from build123d import *

# Parameters (mm, degrees)
SKETCH1_W                      = 19.05
SKETCH1_H                      = 19.05
SKETCH1_W_2                    = 15.875
SKETCH1_H_2                    = 15.875
TUBE_DEPTH                     = 758.9266
SKETCH2_R                      = 2.8956
SIDE_WALL_HOLES_DEPTH          = 20.05
LPATTERN1_COUNT                = 4
LPATTERN1_PITCH                = 210.574466667
CUT_EXTRUDE1_REACH             = 21.05
SKETCH3_R                      = 4.7625
CUT_EXTRUDE1_DIRECTION_2_DEPTH = 1


with BuildPart() as part:
    # Sketch1 → Tube (new body)
    with BuildSketch(Plane(origin=(0, 0, 0), x_dir=(1, 0, 0), z_dir=(0, 1, 0))):
        Rectangle(SKETCH1_W, SKETCH1_H)
        Rectangle(SKETCH1_W_2, SKETCH1_H_2, mode=Mode.SUBTRACT)
    extrude(amount=TUBE_DEPTH)

    # Sketch2 → Side Wall Holes (cut, through all)
    with BuildSketch(Plane.XY.offset(9.525)):
        with Locations((0, 695.325)):
            Circle(SKETCH2_R)
    side_wall_holes = extrude(amount=-SIDE_WALL_HOLES_DEPTH, mode=Mode.SUBTRACT)

    # LPattern1: Side Wall Holes ×4
    with Locations(*[(0, -i * LPATTERN1_PITCH, 0) for i in range(1, LPATTERN1_COUNT)]):
        add(side_wall_holes, mode=Mode.SUBTRACT)

    # Sketch3 → Cut-Extrude1 (cut, up to next)
    with BuildSketch(Plane.ZY.offset(9.525), mode=Mode.PRIVATE) as cut_extrude1_sk1:
        with Locations((0, 674.37)):
            Circle(SKETCH3_R)
    cut_extrude1_tool1 = extrude(cut_extrude1_sk1.sketch, amount=-CUT_EXTRUDE1_REACH, mode=Mode.PRIVATE) & part.part
    add(cut_extrude1_tool1.solids().sort_by_distance((-9.525, 674.37, 0))[0], mode=Mode.SUBTRACT)
    # Sketch3 → Cut-Extrude1 (cut, up to next)
    with BuildSketch(Plane.ZY.offset(9.525), mode=Mode.PRIVATE) as cut_extrude1_sk2:
        with Locations((0, 84.5566)):
            Circle(SKETCH3_R)
    cut_extrude1_tool2 = extrude(cut_extrude1_sk2.sketch, amount=-CUT_EXTRUDE1_REACH, mode=Mode.PRIVATE) & part.part
    add(cut_extrude1_tool2.solids().sort_by_distance((-9.525, 84.5566, 0))[0], mode=Mode.SUBTRACT)

    # Sketch3 → Cut-Extrude1 direction 2 (cut)
    with BuildSketch(Plane.ZY.offset(9.525)):
        with Locations((0, 674.37)):
            Circle(SKETCH3_R)
        with Locations((0, 84.5566)):
            Circle(SKETCH3_R)
    extrude(amount=CUT_EXTRUDE1_DIRECTION_2_DEPTH, mode=Mode.SUBTRACT)


solid = part.part
CAD build for the part. Positions are in the model's coordinates, mm. A direction names the side the tool comes from. Give positions to 0.01 mm unless a question says otherwise; leave off trailing zeros. Write each loop counter-clockwise with the first axis right and the second up, starting at its lowest first coordinate (ties: lowest second). Pieces come first, ordered by that corner, then holes. Notation, with made-up numbers: M 11.25,54 L 70.25,54 A19 cw 70.25,67 Z; hole C -37,-18.75 d6. An arc over 180 degrees is marked long. Put each result on its own line as item: value. Start each with the question number.
(1) Band-saw the part on A-A, the plane y = 145.5. Write the cut outline in (x, z) (1 decimal).
(2) Which spindle directions (+Z, -Z, +X, -X, +Y, -Y) get a long thin tool onto all of the face, cutting with end or side? Do faces 4 (the face through (9.525, 374, 0)), 5 (the face through (7.938, 374, 0)). Say none if no direction does.
(3) Probe L1, parallel to Y at x = 0, z = 9.25; L2, parallel to Y at x = -8.3, z = 0; L3, parallel to Z at x = -2.5, y = 534 (1 decimal). List the from-to ranges inside material, lowest first.
(4) Flat gauge pins, fed straight in: pin 1 Ø4 at (x, z) = (-4, 6.5) entering from -Y; pin 2 Ø5 at (x, z) = (5, 4.5) entering from +Y; pin 3 Ø8.5 at (y, z) = (674.37, 0) entering from -X. Where does each tip first touch, or does it go through?
(5) Mould opens along X. For faces 1 (the face through (-9.525, 374, 0)), 2 (the face through (-9, 0, 0)), 3 (the face through (0, 374, 7.938)) say: +X half, -X half, draft (parallel to the pull), parting line (faces both ways), or undercut.
(6) Band-saw the part on C-C, the plane x = 0. Give the number of separate pieces and of enclosed holes in the cut face, and give its area (3 significant figures).
(7) Band-saw the part on B-B, the plane z = 0. Write the cut outline in (x, y) (1 decimal), and give its area (3 significant figures).
Response values:
1. outline: M -9.5,-9.5 L 9.5,-9.5 L 9.5,9.5 L -9.5,9.5 Z; hole M -7.9,-7.9 L 7.9,-7.9 L 7.9,7.9 L -7.9,7.9 Z
2. face 4: +Z, -Z, +X, +Y, -Y
2. face 5: +Y, -Y
3. L1: y = 0 to 60.71, 66.5 to 271.28, 277.07 to 481.85, 487.65 to 692.43, 698.22 to 758.93
3. L2: y = 0 to 79.79, 89.32 to 669.61, 679.13 to 758.93
3. L3: z = -9.5 to -7.9, 7.9 to 9.5
4. pin 1: stops at y = 0
4. pin 2: passes through
4. pin 3: stops at x = 7.94
5. face 1: -X half
5. face 2: draft
5. face 3: undercut
6. separate pieces: 10
6. enclosed holes: 0
6. area: 2,340 mm2
7. outline: M -9.5,0 L -7.9,0 L -7.9,79.8 L -9.5,79.8 Z; M -9.5,89.3 L -7.9,89.3 L -7.9,669.6 L -9.5,669.6 Z; M -9.5,679.1 L -7.9,679.1 L -7.9,758.9 L -9.5,758.9 Z; M 7.9,0 L 9.5,0 L 9.5,758.9 L 7.9,758.9 Z
7. area: 2,380 mm2
